Geometry check sheet. Reference: drawing and pictorial views, mm from the part's lowest x, y, z. Round coordinates to 2 decimals unless told otherwise and drop trailing zeros. Write each loop counter-clockwise with the first axis right and the second up, starting at its lowest first coordinate (ties: lowest second). Pieces come first, ordered by that corner, then holes. Notation, with made-up numbers: (8, 42) - (22, 42) arc R11 ccw to (22, 63) - close; hole circle Ø1 at (57.5, -11.75). An arc over 180 degrees is marked (long way). Return JSON: item names as keys, results as strings.
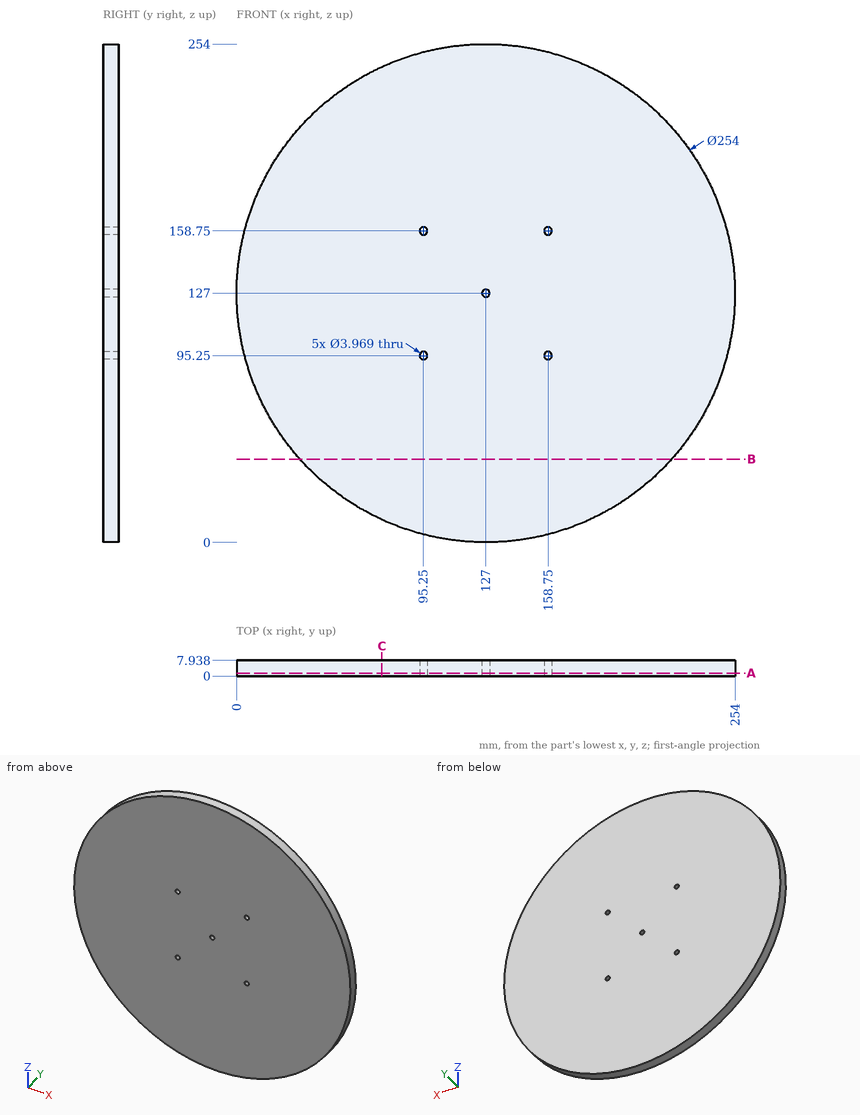
(1) Material ranges on line 1 along X through (y, z) = (3.25, 158.75) (1 decimal); line 2 along X through (y, z) = (5.25, 127) (1 decimal), recorded low to high. Write a range as [from, to].
Response values:
{"line 1": "x = [4, 93.3], [97.2, 156.8], [160.7, 250]", "line 2": "x = [0, 125], [129, 254]"}
(2) Gauge pin test, flat ends, axial feed: pin 1 (4.5 mm diameter, centred on x = 158.75, z = 158.75, fed in from +Y); pin 2 (3 mm diameter, centred on x = 95.25, z = 95.25, fed in from +Y); pin 3 (3 mm diameter, centred on y = 4.5, z = 154.5, fed in from +X). Record the tip position at first contact, or that the pin passes through.
Response values:
{"pin 1": "stops at y = 7.94", "pin 2": "passes through", "pin 3": "stops at x = 251.31"}
(3) Section check A-A, the plane y = 1.5. Give the number of separate pieces and of enclosed holes in the cut face, plus the area to 3 significant figures.
Response values:
{"separate pieces": "1", "enclosed holes": "5", "area": "50,600 mm^2"}
(4) Section check B-B, the plane z = 42.5. Enter the section's corners in (x, y), plus the area to 4 significant figures.
Response values:
{"outline": "(32.19, 0) - (221.81, 0) - (221.81, 7.94) - (32.19, 7.94) - close", "area": "1,505 mm^2"}
(5) Section check C-C, the plane x = 74. Enter the section's corners in (y, z), plus the area to 3 significant figures.
Response values:
{"outline": "(0, 11.59) - (7.94, 11.59) - (7.94, 242.41) - (0, 242.41) - close", "area": "1,830 mm^2"}
